Print and shaded views of the part. All mm, measured from the part's lowest x, y and z. A direction names the side the tool comes from. Round coordinates to 2 decimals unless told otherwise and drop trailing zeros. Write each loop counter-clockwise with the first axis right and the second up, starting at its lowest first coordinate (ties: lowest second). Pieces come first, ordered by that corner, then holes. Notation, with made-up numbers: M 87,11.25 L 129,11.25 A24 ccw 129,35.25 Z; hole C 50.25,60.25 d8. An arc over 180 degrees is marked long. Write item = value, one per line. Start each with the question number.
Q1. Tool access for the marked faces 1 and 2: list every direction of +Z, -Z, +X, -X, +Y, -Y with a clear straight run to the whole face (end or side of a thin tool).
Q2. Drop flat-ended pins along their axis: P1, Ø8, axis at y = 6.5, z = 12.5, coming from the +X side (1 decimal); P2, Ø8.5, axis at x = 44.5, z = 22, coming from the -Y side. Give the stop position or say it passes through.
Q3. Probe L1, parallel to X at y = 13, z = 25.4; L2, parallel to Y at x = 53.5, z = 35; L3, parallel to X at y = 12.25, z = 18. List the from-to ranges inside material, lowest first.
Q4. Band-saw the part on B-B on x = 35. Write the cut outline in (y, z), plus the area to 3 significant figures.
Q5. Band-saw the part on A-A on z = 25.4. Write the cut outline in (x, y), plus the area to 3 significant figures.
Q6. Band-saw the part on C-C on y = 18.5. Write the cut outline in (x, z), plus the area to 3 significant figures.
Q7. Pull direction X, two halves, no side cores. Call the marked faces 3, 4 and 5: released by +X, released by -X, zero draft, split by the parting line, or undercut.
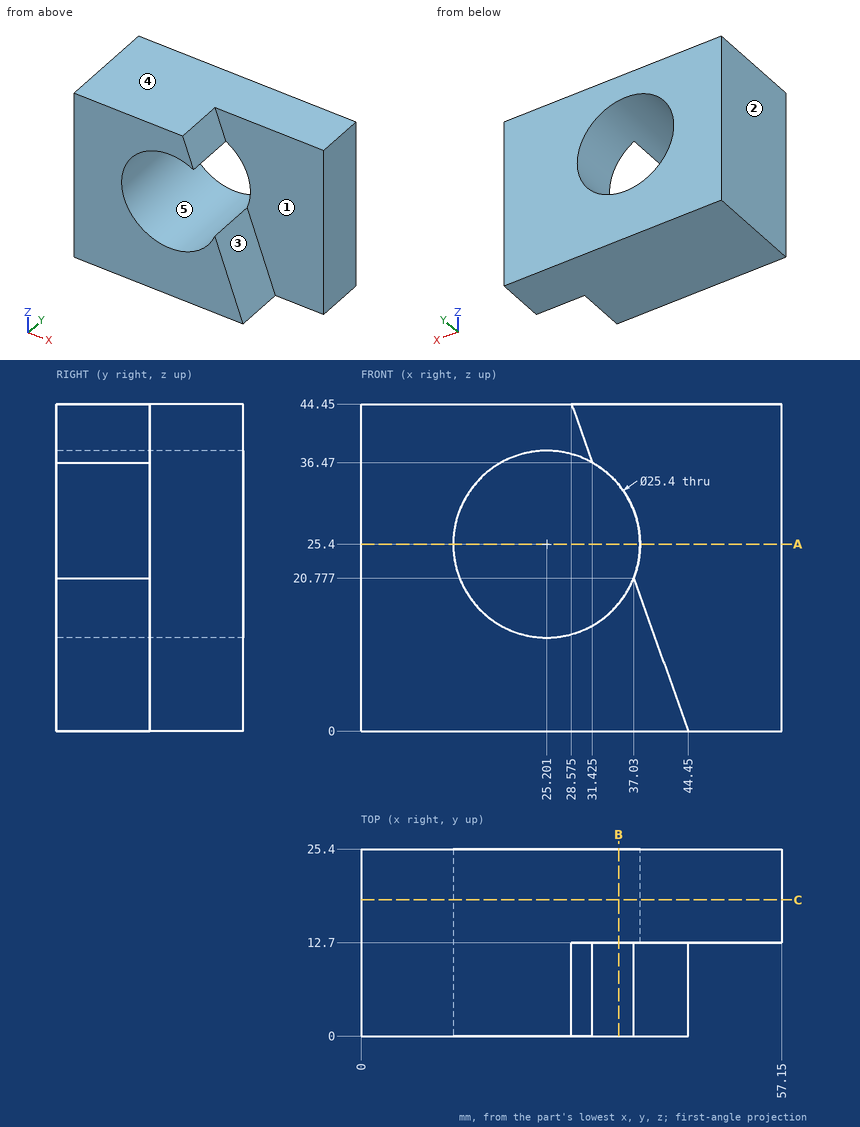
Conclusion:
q1.face_1 = +Z, +X, -Y
q1.face_2 = +Z, -Z, -X, +Y, -Y
q2.P1 = 41.4
q2.P2 = 12.7
q3.L1 = 0 to 12.5, 37.9 to 57.15
q3.L2 = 12.7 to 25.4
q3.L3 = 0 to 14.88, 35.52 to 38.02
q4.outline = M 0,0 L 25.4,0 L 25.4,17.32 L 0,17.32 Z; M 12.7,33.48 L 25.4,33.48 L 25.4,44.45 L 12.7,44.45 Z
q4.area = 579 mm^2
q5.outline = M 0,0 L 12.5,0 L 12.5,25.4 L 0,25.4 Z; M 37.9,12.7 L 57.15,12.7 L 57.15,25.4 L 37.9,25.4 Z
q5.area = 562 mm^2
q6.outline = M 0,0 L 57.15,0 L 57.15,44.45 L 0,44.45 Z; hole C 25.2,25.4 d25.4
q6.area = 2,030 mm^2
q7.face_3 = released by +X
q7.face_4 = zero draft
q7.face_5 = undercut
